Geometry check sheet. Reference: the model listing, model coordinates, mm. A direction names the side the tool comes from. Round coordinates to 2 decimals unless told otherwise and drop trailing zeros. Write each loop counter-clockwise with the first axis right and the second up, starting at its lowest first coordinate (ties: lowest second). Pieces come first, ordered by that corner, then holes.
Item 1: Depth check by flat-ended pin: P1, Ø1, axis at y = -0.5, z = -1, coming from the +X side; P2, Ø1.5, axis at x = 0.5, y = 0, coming from the -Z side. Enter the tip coordinate at first touch or a pass-through.
Item 2: Cross-section at C-C (x = 3). Enter the section's corners in (y, z), then the cut area to 3 significant figures.
Item 3: Scan lines: probe 1 along Y at (x, z) = (2.5, 0.75); probe 2 along Y at (x, z) = (11.5, -0.45); probe 3 along Z at (x, y) = (4.5, -0.2). Record each from-to range of solid material in increasing order.
Item 4: Access from +Z, -Z, +X, -X, +Y, -Y to the whole of each face (thin tool, end or side, straight path). Record for faces 1 (the face through (-1.5, 0, 0)), 2 (the face through (6.66, 0.27, -0.86)).
Item 5: Cross-section at A-A (z = 0). Enter the section's corners in (x, y).
from build123d import *

# Parameters (mm, degrees)
SKETCH1_R           = 0.9
BOSS_EXTRUDE1_DEPTH = 14
SKETCH2_R           = 1.5
BOSS_EXTRUDE2_DEPTH = 1.5
CHAMFER1_SIZE       = 0.5


with BuildPart() as part:
    # Sketch1 → Boss-Extrude1 (new body)
    with BuildSketch(Plane(origin=(0, 0, 0), x_dir=(0, 0, -1), z_dir=(1, 0, 0))):
        Circle(SKETCH1_R)
    extrude(amount=BOSS_EXTRUDE1_DEPTH)

    # Sketch2 → Boss-Extrude2 (add)
    with BuildSketch(Plane(origin=(0, 0, 0), x_dir=(0, 0, -1), z_dir=(1, 0, 0))):
        Circle(SKETCH2_R)
    extrude(amount=-BOSS_EXTRUDE2_DEPTH)

    # Chamfer1
    chamfer1_edges = [part.edges().sort_by_distance(p)[0] for p in [
        (14, 0, 0.9),
        (0, 0, 1.5),
    ]]
    chamfer(chamfer1_edges, length=CHAMFER1_SIZE)


solid = part.part
Resolved:
1. P1: stops at x = 13.78
1. P2: stops at z = -1.25
2. outline: circle Ø1.8 at (0, 0)
2. area: 2.54 mm2
3. probe 1: y = -0.5 to 0.5
3. probe 2: y = -0.78 to 0.78
3. probe 3: z = -0.88 to 0.88
4. face 1: +Z, -Z, -X, +Y, -Y
4. face 2: +X
5. outline: (-1.5, -1.5) - (-0.5, -1.5) - (0, -1) - (0, -0.9) - (13.5, -0.9) - (14, -0.4) - (14, 0.4) - (13.5, 0.9) - (0, 0.9) - (0, 1) - (-0.5, 1.5) - (-1.5, 1.5) - close
